Verification items for the finished model (mm, model axes). Give positions to 0.01 mm unless a question says otherwise; leave off trailing zeros. Loops run counter-clockwise (first coordinate to the right, second up) from the corner with the lowest first, then second, coordinate; pieces in that order, holes last. Notation, with made-up numbers: (-33, -2.75) - (25, -2.75) arc R13 cw to (25, 16.25) - close; hole circle Ø3 at (-30, 82). An arc over 180 degrees is marked (long way). Use one line per item in the form item = value.
```python
from build123d import *

# Parameters (mm, degrees)
F1_DEPTH = 38.1
F2_DEPTH = 38.1


with BuildPart() as f1:
    # F0 (on Top) → F1 (new body)
    with BuildSketch(Plane.XY):
        with BuildLine():
            Line((304.8, -287.3375), (304.8, 287.3375))
            Line((304.8, 287.3375), (203.2, 287.3375))
            ThreePointArc((203.2, 287.3375), (165.1, 249.2375), (127, 287.3375))
            Line((127, 287.3375), (-304.8, 287.3375))
            Line((-304.8, 287.3375), (-304.8, -287.3375))
            Line((-304.8, -287.3375), (304.8, -287.3375))
        make_face()
        with BuildLine():
            ThreePointArc((127, 287.3375), (165.1, 249.2375), (203.2, 287.3375))
            Line((203.2, 287.3375), (127, 287.3375))
        make_face()
    extrude(amount=F1_DEPTH)

    # F0 (on Top) → F2 (cut)
    with BuildSketch(Plane.XY):
        with BuildLine():
            ThreePointArc((127, 287.3375), (165.1, 249.2375), (203.2, 287.3375))
            Line((203.2, 287.3375), (127, 287.3375))
        make_face()
    extrude(amount=F2_DEPTH, mode=Mode.SUBTRACT)


solid = f1.part
```
1. Scan lines: probe 1 along Y at (x, z) = (172.5, 20.5); probe 2 along Y at (x, z) = (141, 27). Record each from-to range of solid material in increasing order.
Result set:
probe_1 = -287.34 to 249.96
probe_2 = -287.34 to 257.83
2. Depth check by flat-ended pin: pin 1 Ø6 at (x, z) = (184, 23.5) entering from +Y. Enter the tip coordinate at first touch or a pass-through.
Result set:
pin_1 = 256.16
3. Section check A-A, the plane x = 165.1. Record the cut outline in (y, z), then the cut area to 3 significant figures.
Result set:
outline = (-287.34, 0) - (249.24, 0) - (249.24, 38.1) - (-287.34, 38.1) - close
area = 20,400 mm²
